Verification items for the finished model (mm, model axes). A direction names the side the tool comes from. Give positions to 0.01 mm unless a question says otherwise; leave off trailing zeros. Order: outer loops, then holes, each group sorted by start corner. A loop starts at its lowest first (then second) coordinate and runs counter-clockwise, first axis right, second up. Notation, with made-up numbers: (61, -10.5) -> (85, -10.5) arc R34 cw to (85, 25.5) -> close; hole circle Ø7 at (35, 45.25). An arc over 180 degrees is marked (long way). Return JSON: item names as keys, results as strings. Group by question number.
(1) Release check for a two-part mould opening along X. For faces 1 (the face through (84.2, 1.77, -20.15)), 2 (the face through (5.742, 2.254, -11.234)), 3 (the face through (81, 2.25, -13.04)), 4 (the face through (0, 2, -13)) record: pulls with the +X half, pulls with the -X half, needs draft (parallel to the pull), parting line crosses it, or undercut.
(2) Cross-section at A-A on z = -12.7. Enter the section's corners in (x, y) (1 decimal), then the cut area to 3 significant figures.
(3) Tool access check on faces 5 (the face through (88.9, 2, -13)), 6 (the face through (84.2, 1.77, -7.45)). Record the directions out of +Z, -Z, +X, -X, +Y, -Y that give a thin tool (end or side, any length) a straight path to the whole face; none if there is none.
(4) Depth check by flat-ended pin: pin 1 Ø2 at (x, z) = (76.5, -17) entering from -Y; pin 2 Ø2.5 at (x, z) = (6.35, -12.7) entering from +Y. Enter the tip coordinate at first touch or a pass-through.
(5) Cross-section at C-C on z = -19.05. Enter the section's corners in (x, y) (3 decimals), then the cut area to 3 significant figures.
(6) Thickness scan on line 1 along X through (y, z) = (1, -12.7); line 2 along Y through (x, z) = (82.25, -6.35) (3 decimals); line 3 along Z through (x, y) = (82.55, 1.75). Record the ranges inside material, lowest first.
(7) Cross-section at B-B on x = 6.35. Enter the section's corners in (y, z) (1 decimal), then the cut area to 3 significant figures.
from build123d import *

# Parameters (mm, degrees)
SKETCH1_W           = 88.9
SKETCH1_H           = 25.4
BOSS_EXTRUDE1_DEPTH = 4.445
SKETCH3_R           = 1.190625
CUT_EXTRUDE2_DEPTH  = 9.525
SKETCH4_R           = 1.5875
CUT_EXTRUDE3_DEPTH  = 93.564183273


with BuildPart() as part:
    # Sketch1 → Boss-Extrude1 (new body)
    with BuildSketch(Plane(origin=(0, 0, 0), x_dir=(1, 0, 0), z_dir=(0, 1, 0))):
        with Locations((44.45, 12.7)):
            Rectangle(SKETCH1_W, SKETCH1_H)
    extrude(amount=BOSS_EXTRUDE1_DEPTH)

    # Sketch3 → Cut-Extrude2 (cut)
    with BuildSketch(Plane(origin=(88.9, 0, 0), x_dir=(0, 0, -1), z_dir=(1, 0, 0))):
        with Locations((19.05, 2.2225)):
            Circle(SKETCH3_R)
        with Locations((6.35, 2.2225)):
            Circle(SKETCH3_R)
    extrude(amount=-CUT_EXTRUDE2_DEPTH, mode=Mode.SUBTRACT)

    # Sketch4 → Cut-Extrude3 (cut, through all)
    with BuildSketch(Plane(origin=(0, 4.445, 0), x_dir=(1, 0, 0), z_dir=(0, 1, 0))):
        with Locations(Location((6.35, 12.7, 0), (0, 0, 270))):
            Circle(SKETCH4_R)
        with Locations(Location((82.55, 12.7, 0), (0, 0, 270))):
            Circle(SKETCH4_R)
    extrude(amount=-CUT_EXTRUDE3_DEPTH, mode=Mode.SUBTRACT)


solid = part.part
Verdict:
{
 "1": {"face 1": "needs draft", "face 2": "undercut", "face 3": "undercut", "face 4": "pulls with the -X half"},
 "2": {"outline": "(0, 0) -> (4.8, 0) -> (4.8, 4.4) -> (0, 4.4) -> close; (7.9, 0) -> (81, 0) -> (81, 4.4) -> (7.9, 4.4) -> close; (84.1, 0) -> (88.9, 0) -> (88.9, 4.4) -> (84.1, 4.4) -> close", "area": "367 mm²"},
 "3": {"face 5": "+Z, -Z, +X, +Y, -Y", "face 6": "+X"},
 "4": {"pin 1": "y = 0", "pin 2": "through"},
 "5": {"outline": "(0, 0) -> (88.9, 0) -> (88.9, 1.032) -> (79.375, 1.032) -> (79.375, 3.413) -> (88.9, 3.413) -> (88.9, 4.445) -> (0, 4.445) -> close", "area": "372 mm²"},
 "6": {"line 1": "0 to 4.76, 7.94 to 80.96, 84.14 to 88.9", "line 2": "0 to 1.032, 3.413 to 4.445", "line 3": "-25.4 to -20.14, -17.96 to -14.29, -11.11 to -7.44, -5.26 to 0"},
 "7": {"outline": "(0, -25.4) -> (4.4, -25.4) -> (4.4, -14.3) -> (0, -14.3) -> close; (0, -11.1) -> (4.4, -11.1) -> (4.4, 0) -> (0, 0) -> close", "area": "98.8 mm²"}
}
